```python
from build123d import *

# Parameters (mm, degrees)
SKETCH1_W           = 16.9901
SKETCH1_H           = 11.326733
BOSS_EXTRUDE1_DEPTH = 1
SKETCH2_W           = 12.826733
SKETCH2_H           = 6.1267257
BOSS_EXTRUDE2_DEPTH = 0.15
FILLET2_R           = 0.1
SKETCH3_W           = 6.250546152
SKETCH3_H           = 4.820472611
SKETCH3_W_2         = 2.746840533
SKETCH3_H_2         = 3.904582815
SKETCH3_W_3         = 3.692789168
BOSS_EXTRUDE3_DEPTH = 5
BOSS_EXTRUDE4_DEPTH = 2


with BuildPart() as part:
    # Sketch1 → Boss-Extrude1 (new body)
    with BuildSketch(Plane(origin=(0, 0, 0), x_dir=(1, 0, 0), z_dir=(0, 1, 0))):
        with Locations((8.49505, -5.6633665)):
            Rectangle(SKETCH1_W, SKETCH1_H)
    extrude(amount=BOSS_EXTRUDE1_DEPTH)

    # Sketch2 → Boss-Extrude2 (add)
    with BuildSketch(Plane(origin=(16.9901, 0, 0), x_dir=(0, 0, -1), z_dir=(1, 0, 0))):
        with Locations((-5.6633665, 3.06336285)):
            Rectangle(SKETCH2_W, SKETCH2_H)
    extrude(amount=BOSS_EXTRUDE2_DEPTH)

    # Fillet2
    fillet2_edges = [part.edges().sort_by_distance(p)[0] for p in [
        (17.0651, 6.1267257, 12.076733),
        (17.0651, 0, 12.076733),
        (17.0651, 0, -0.75),
        (17.0651, 6.1267257, -0.75),
    ]]
    fillet(fillet2_edges, radius=FILLET2_R)

    # Sketch3 → Boss-Extrude3 (add)
    with BuildSketch(Plane(origin=(0, 1, 0), x_dir=(1, 0, 0), z_dir=(0, 1, 0))):
        Polygon((6.971259917, -6.145413761), (12.546939904, -6.145413761), (12.546939904, -8.716332487), (11.165071089, -8.716332487), (11.165071089, -10.965886372), (6.971259917, -10.965886372), align=None)
        with Locations((3.492485517, -8.555650067)):
            Rectangle(SKETCH3_W, SKETCH3_H)
        Polygon((16.853228769, -6.145413761), (14.925039725, -6.145413761), (13.864535751, -8.925219633), (11.550708898, -8.925219633), (11.550708898, -10.965886372), (16.853228769, -10.965886372), align=None)
        Polygon((16.853228769, -0.409051354), (16.853228769, -4.313634169), (16.451522719, -4.313634169), (16.451522719, -5.149182755), (16.001611942, -5.454479354), (14.748289063, -5.454479354), (14.541123514, -5.149182755), (14.541123514, -4.313634169), (14.057354655, -4.313634169), (14.057354655, -5.149182755), (13.68878146, -5.399285995), (12.145233853, -5.399285995), (10.709853969, -5.399285995), (10.459750729, -5.149182755), (10.459750729, -4.313634169), (10.088036395, -4.313634169), (10.088036395, -0.409051354), align=None)
        with Locations((8.344680184, -2.361342761)):
            Rectangle(SKETCH3_W_2, SKETCH3_H_2)
        with Locations((4.771364009, -2.361342761)):
            Rectangle(SKETCH3_W_3, SKETCH3_H_2)
    extrude(amount=BOSS_EXTRUDE3_DEPTH)

    # Sketch4 → Boss-Extrude4 (add)
    with BuildSketch(Plane(origin=(0, 1, 0), x_dir=(1, 0, 0), z_dir=(0, 1, 0))):
        Polygon((0.367212441, -4.313634169), (0.367212441, -0.409051354), (1.636603562, -0.409051354), (2.664971052, -1.437418845), (2.664971052, -4.313634169), align=None)
    extrude(amount=BOSS_EXTRUDE4_DEPTH)


solid = part.part
```
Geometry check sheet. Reference: the model listing, model coordinates, mm. A direction names the side the tool comes from. Coordinates: 2 decimals unless noted, no trailing zeros. Write each loop counter-clockwise with the first axis right and the second up, starting at its lowest first coordinate (ties: lowest second). Pieces come first, ordered by that corner, then holes. Notation, with made-up numbers: M 64,70.25 L 83,70.25 A25 cw 83,98.25 Z; hole C 25,35.25 d11. An arc over 180 degrees is marked long. Use one line per item in the form item = value. Start each with the question number.
1) Set-up check for faces 4 (the flat face through (5, 3, 0.409)), 5 (the flat face through (9, 3, 10.966)), 6 (the flat face through (2.665, 2, 3)), 7 (the flat face through (12, 3, 8.716)), 8 (the flat face through (10, 6, 9)): record each of +Z, -Z, +X, -X, +Y, -Y from which the full face is reachable in a straight line by a thin tool's end or side.
2) Section check B-B on x = 6.25. Enter the section's corners in (y, z), and give its area (3 significant figures).
3) Section check A-A on z = 1.75. Enter the section's corners in (x, y).
4) Release check for a two-part mould opening along X. For faces 1 (the flat face through (8, 6, 2)), 2 (the flat face through (10.46, 3.5, 4.7)), 3 (the flat face through (9.718, 3, 2)) record: pulls with the +X half, pulls with the -X half, needs draft (parallel to the pull), parting line crosses it, or undercut.
5) Section check C-C on y = 2. State how many separate pieces and enclosed holes the cut face has, and give its area (3 significant figures).
6) Go/stop test with flat-tipped pins: pin 1 Ø3 at (x, y) = (5, 4) entering from -Z; pin 2 Ø2.5 at (x, z) = (2.5, 7.5) entering from +Y; pin 3 Ø1.6 at (y, z) = (4.5, 10) entering from -X. Record where each tip stops, or that it passes through.
7) Thickness scan on probe 1 along Z at (x, y) = (6.5, 4); probe 2 along Z at (x, y) = (16, 3.75); probe 3 along Y at (x, z) = (1, 2.25). Record the ranges inside material, lowest first. Write a range as from..to.
Responses:
q1.face_4 = -Z, -X, +Y
q1.face_5 = +Z, -X, +Y
q1.face_6 = -Z, +Y
q1.face_7 = +Y
q1.face_8 = +Z, -Z, -X, +Y
q2.outline = M 0,0 L 1,0 L 1,0.41 L 6,0.41 L 6,4.31 L 1,4.31 L 1,6.15 L 6,6.15 L 6,10.97 L 1,10.97 L 1,11.33 L 0,11.33 Z
q2.area = 55.0 mm2
q3.outline = M 0,0 L 17.14,0 L 17.14,6.13 L 16.99,6.13 L 16.99,1 L 16.85,1 L 16.85,6 L 10.09,6 L 10.09,1 L 9.72,1 L 9.72,6 L 6.97,6 L 6.97,1 L 6.62,1 L 6.62,6 L 2.92,6 L 2.92,1 L 2.66,1 L 2.66,3 L 0.37,3 L 0.37,1 L 0,1 Z
q4.face_1 = needs draft
q4.face_2 = pulls with the -X half
q4.face_3 = undercut
q5.separate_pieces = 8
q5.enclosed_holes = 0
q5.area = 139 mm2
q6.pin_1 = 0.41
q6.pin_2 = 6
q6.pin_3 = 0.37
q7.probe_1 = 0.41..4.31, 6.15..10.97
q7.probe_2 = 0.41..5.45, 6.15..10.97
q7.probe_3 = 0..3
